Work out the finished part from the listing and answer in its coordinate system (mm). Face numbers are marked on the shaded views. A direction names the side the tool comes from. Round coordinates to 2 decimals unless told otherwise and drop trailing zeros. Order: outer loops, then holes, each group sorted by start corner. A loop starts at its lowest first (then second) coordinate and runs counter-clockwise, first axis right, second up. Notation, with made-up numbers: (16.5, -33) - (43.5, -33) arc R36 ccw to (43.5, 1) - close; hole circle Ø6 at (16.5, -2). An arc over 180 degrees is marked (long way). Use CSV: the item, a comma, the result in double quotes.
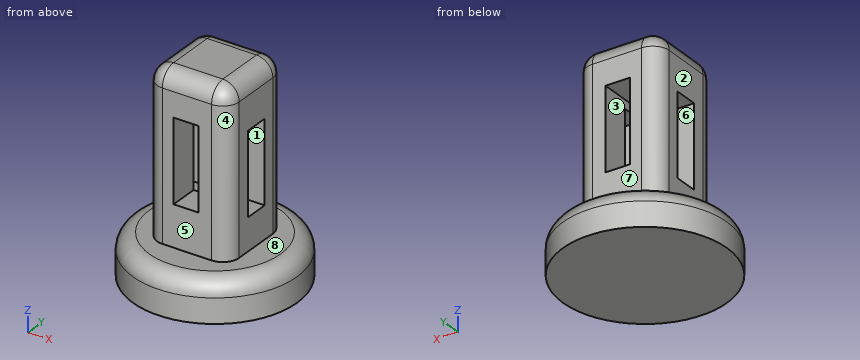
from build123d import *

# Parameters (mm, degrees)
F0_R     = 25.4
F1_DEPTH = 12.7
F2_W     = 25.4
F2_H     = 25.4
F3_DEPTH = 50.8
F4_R     = 5.08
F5_W     = 7.62
F5_H     = 25.4
F6_DEPTH = 25.4
F7_W     = 7.62
F7_H     = 25.4
F8_DEPTH = 25.4


with BuildPart() as f1:
    # F0 (on Top) → F1 (new body)
    with BuildSketch(Plane.XY):
        Circle(F0_R)
    extrude(amount=F1_DEPTH)

    # F2 (on face) → F3 (join)
    with BuildSketch(Plane.XY.offset(12.7)):
        Rectangle(F2_W, F2_H)
    extrude(amount=F3_DEPTH)

    # F4
    f4_edges = [f1.edges().sort_by_distance(p)[0] for p in [
        (12.7, -12.7, 38.1),
        (-12.7, -12.7, 38.1),
        (12.7, 12.7, 38.1),
        (-12.7, 12.7, 38.1),
        (-25.4, 0, 12.7),
        (-12.7, 0, 63.5),
        (0, -12.7, 63.5),
        (12.7, 0, 63.5),
        (0, 12.7, 63.5),
    ]]
    fillet(f4_edges, radius=F4_R)

    # F5 (on face) → F6 (cut)
    with BuildSketch(Plane.YZ.offset(12.7)):
        with Locations((0.143903, 35.440086)):
            Rectangle(F5_W, F5_H)
    extrude(amount=-F6_DEPTH, mode=Mode.SUBTRACT)

    # F7 (on face) → F8 (cut)
    with BuildSketch(Plane(origin=(0, 12.7, 0), x_dir=(-1, 0, 0), z_dir=(0, 1, 0))):
        with Locations((0.287806, 38.145431)):
            Rectangle(F7_W, F7_H)
    extrude(amount=-F8_DEPTH, mode=Mode.SUBTRACT)


solid = f1.part
(1) The mould has two halves that part along Y. Classify the marked faces 5, 6, 7 and 8: released by +Y, released by -Y, zero draft, split by the parting line, or undercut.
Findings below:
face 5,"released by -Y"
face 6,"undercut"
face 7,"released by +Y"
face 8,"zero draft"
(2) Find the intervals of material crossed by L1, parallel to Z at x = 1, y = -1; L2, parallel to X at y = 7, z = 49; L3, parallel to Z at x = -1, y = -15.5, in increasing order. Write a range as from..to.
Findings below:
L1,"z = 0..22.74, 50.85..63.5"
L2,"x = -12.7..-4.1, 3.52..12.7"
L3,"z = 0..12.7"
(3) Find section D-D (z = 53). Determine the outline of the cut face in (x, y).
Findings below:
outline,"(-12.7, -7.62) arc R5.08 ccw to (-7.62, -12.7) - (7.62, -12.7) arc R5.08 ccw to (12.7, -7.62) - (12.7, 7.62) arc R5.08 ccw to (7.62, 12.7) - (-7.62, 12.7) arc R5.08 ccw to (-12.7, 7.62) - close"
(4) Each of these flat-tipped pins is pushed along its axis until it touches: pin 1 (17 mm diameter, centred on y = 3.5, z = 32, fed in from -X); pin 2 (2 mm diameter, centred on x = -18, y = 7.5, fed in from -Z); pin 3 (1 mm diameter, centred on y = 4.5, z = 12, fed in from -X); pin 4 (3 mm diameter, centred on y = -13.5, z = 8.5, fed in from -X). Where does it stop, or does it pass through?
Findings below:
pin 1,"stops at x = -12.7"
pin 2,"stops at z = 0"
pin 3,"stops at x = -23.17"
pin 4,"stops at x = -22.33"
(5) For the marked faces 1, 2, 3 and 4, determine the directions among +Z, -Z, +X, -X, +Y, -Y from which every point of the face is accessible in a straight line to the end or side of a thin tool.
Findings below:
face 1,"+X, -X"
face 2,"+Z, -X, +Y, -Y"
face 3,"+Y, -Y"
face 4,"+Z, +X, -Y"
(6) Find section A-A (y = 0). Determine the outline of the cut face in (x, z), and give its area (3 significant figures).
Findings below:
outline,"(-25.4, 0) - (25.4, 0) - (25.4, 7.62) arc R5.08 ccw to (20.32, 12.7) - (12.7, 12.7) - (12.7, 22.74) - (-12.7, 22.74) - (-12.7, 12.7) - (-20.32, 12.7) arc R5.08 ccw to (-25.4, 7.62) - close; (-12.7, 48.14) - (-4.1, 48.14) - (-4.1, 50.85) - (3.52, 50.85) - (3.52, 48.14) - (12.7, 48.14) - (12.7, 58.42) arc R5.08 ccw to (7.62, 63.5) - (-7.62, 63.5) arc R5.08 ccw to (-12.7, 58.42) - close"
area,"1,250 mm²"
(7) Find section C-C (z = 28). Determine the outline of the cut face in (x, y), and give its area (3 significant figures).
Findings below:
outline,"(-12.7, -7.62) arc R5.08 ccw to (-7.62, -12.7) - (-4.1, -12.7) - (-4.1, -3.67) - (-12.7, -3.67) - close; (-12.7, 3.95) - (-4.1, 3.95) - (-4.1, 12.7) - (-7.62, 12.7) arc R5.08 ccw to (-12.7, 7.62) - close; (3.52, -12.7) - (7.62, -12.7) arc R5.08 ccw to (12.7, -7.62) - (12.7, -3.67) - (3.52, -3.67) - close; (3.52, 3.95) - (12.7, 3.95) - (12.7, 7.62) arc R5.08 ccw to (7.62, 12.7) - (3.52, 12.7) - close"
area,"294 mm²"
(8) Find section B-B (x = 0). Determine the outline of the cut face in (y, z), and give its area (3 significant figures).
Findings below:
outline,"(-25.4, 0) - (25.4, 0) - (25.4, 7.62) arc R5.08 ccw to (20.32, 12.7) - (12.7, 12.7) - (12.7, 25.45) - (3.95, 25.45) - (3.95, 22.74) - (-3.67, 22.74) - (-3.67, 25.45) - (-12.7, 25.45) - (-12.7, 12.7) - (-20.32, 12.7) arc R5.08 ccw to (-25.4, 7.62) - close; (-12.7, 50.85) - (12.7, 50.85) - (12.7, 58.42) arc R5.08 ccw to (7.62, 63.5) - (-7.62, 63.5) arc R5.08 ccw to (-12.7, 58.42) - close"
area,"1,250 mm²"
